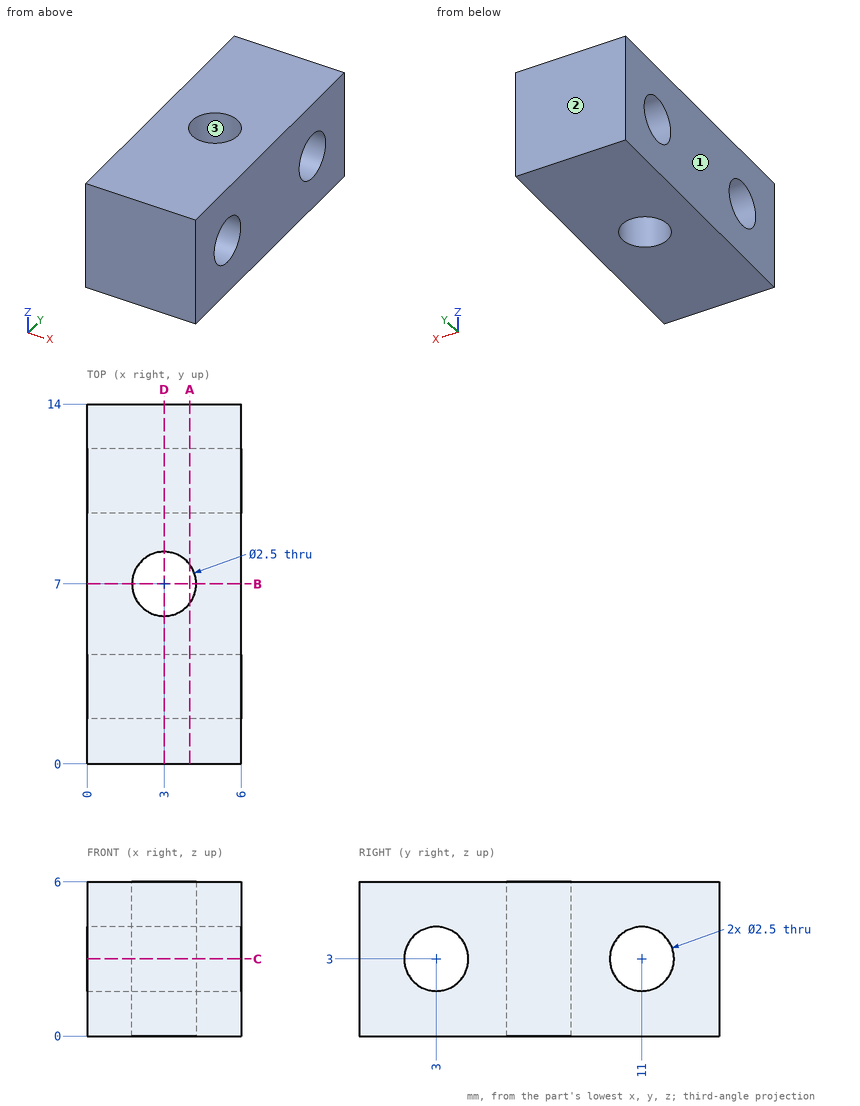
Could you check a few things on this drawing? It's one solid part, dimensions in mm from its lowest x, y, z. Coordinates: 2 decimals unless noted, no trailing zeros. Order: outer loops, then holes, each group sorted by start corner. A loop starts at its lowest first (then second) coordinate and runs counter-clockwise, first axis right, second up.
1. Thinking about a two-plate mould opening in X: for the marked faces 1, 2 and 3, which applies, +X half, -X half, draft (parallel to the pull), parting line (faces both ways), or undercut?
2. I need wall thicknesses on line 1 (Y direction, x = 1.05, z = 2.15); line 2 (Y direction, x = 5.35, z = 2.75); line 3 (Y direction, x = 3.1, z = 3). Which ranges of each line are inside material? Lowest first, please.
3. I'm going to push a flat-ended pin straight in: pin 1 (2 mm diameter, centred on y = 11, z = 3, fed in from -X). Where does the tip first touch, or does it pass through?
4. If we section it at B-B (y = 7): Please give me the cut outline in (x, z).
5. If we section it at D-D (x = 3): Please give me the cut outline in (y, z), then the cut area to 3 significant figures.
6. If we section it at A-A (x = 4): Please give me the cut outline in (y, z), then the cut area to 3 significant figures.
7. If we section it at C-C (z = 3): Please give me the cut outline in (x, y).
Entries:
1. face 1: -X half
1. face 2: draft
1. face 3: undercut
2. line 1: y = 0 to 2.08, 3.92 to 10.08, 11.92 to 14
2. line 2: y = 0 to 1.78, 4.22 to 9.78, 12.22 to 14
2. line 3: y = 0 to 1.75, 4.25 to 5.75, 8.25 to 9.75, 12.25 to 14
3. pin 1: passes through
4. outline: (0, 0) - (1.75, 0) - (1.75, 6) - (0, 6) - close; (4.25, 0) - (6, 0) - (6, 6) - (4.25, 6) - close
5. outline: (0, 0) - (5.75, 0) - (5.75, 6) - (0, 6) - close; (8.25, 0) - (14, 0) - (14, 6) - (8.25, 6) - close; hole circle Ø2.5 at (3, 3); hole circle Ø2.5 at (11, 3)
5. area: 59.2 mm2
6. outline: (0, 0) - (6.25, 0) - (6.25, 6) - (0, 6) - close; (7.75, 0) - (14, 0) - (14, 6) - (7.75, 6) - close; hole circle Ø2.5 at (3, 3); hole circle Ø2.5 at (11, 3)
6. area: 65.2 mm2
7. outline: (0, 0) - (6, 0) - (6, 1.75) - (0, 1.75) - close; (0, 4.25) - (6, 4.25) - (6, 9.75) - (0, 9.75) - close; (0, 12.25) - (6, 12.25) - (6, 14) - (0, 14) - close; hole circle Ø2.5 at (3, 7)
